Source: CAD feature listing. Evaluate the final solid. Frame: model axes, mm. Face numbers are marked on the shaded views. A direction names the side the tool comes from. Give positions to 0.01 mm unless a question says otherwise; leave off trailing zeros. Order: outer loops, then holes, each group sorted by start corner. A loop starts at its lowest first (then second) coordinate and runs counter-clockwise, first axis right, second up. Notation, with made-up numbers: (71, 33) -> (122, 33) arc R29 ccw to (122, 64) -> close; hole circle Ø7 at (37.5, -21). An arc over 180 degrees is marked (long way). Use CSV: the item, a comma, the result in double quotes.
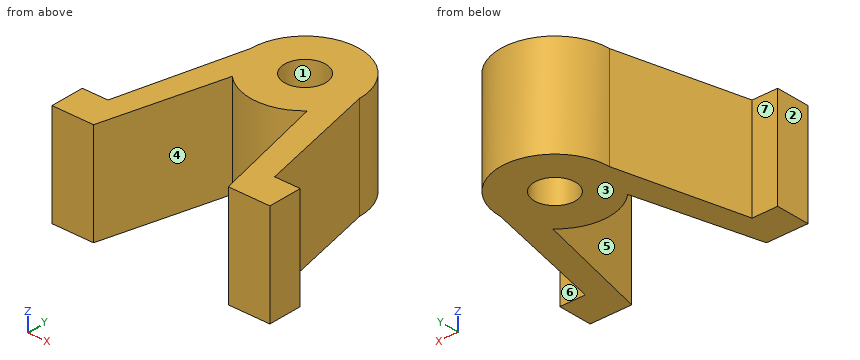
```python
from build123d import *

# Parameters (mm, degrees)
SKETCH_1_R      = 4
EXTRUDE_1_DEPTH = 20


with BuildPart() as part:
    # 草图1 → 凸台-拉伸1 (new body)
    with BuildSketch(Plane.XY):
        with BuildLine():
            Line((-37.719289559, 36.699716541), (-32.049702854, 11.94104698))
            Line((-32.049702854, 11.94104698), (-27.049702854, 11.94104698))
            Line((-27.049702854, 11.94104698), (-27.049702854, 5.329716541))
            Line((-27.049702854, 5.329716541), (-35.173631719, 5.329716541))
            Line((-35.173631719, 5.329716541), (-41.015175762, 29.009348728))
            ThreePointArc((-41.015175762, 29.009348728), (-48.339289559, 26.079716541), (-55.663403355, 29.009348728))
            Line((-55.663403355, 29.009348728), (-61.504947398, 5.329716541))
            Line((-61.504947398, 5.329716541), (-69.628876263, 5.329716541))
            Line((-69.628876263, 5.329716541), (-69.628876263, 11.94104698))
            Line((-69.628876263, 11.94104698), (-64.628876263, 11.94104698))
            Line((-64.628876263, 11.94104698), (-58.959289559, 36.699716541))
            ThreePointArc((-58.959289559, 36.699716541), (-48.339289559, 47.319716541), (-37.719289559, 36.699716541))
        make_face()
        with Locations((-48.339289559, 36.699716541)):
            Circle(SKETCH_1_R, mode=Mode.SUBTRACT)
    extrude(amount=EXTRUDE_1_DEPTH)


solid = part.part
```
1. Ray query, line 1 along X through (y, z) = (27.5, 9); line 2 along X through (y, z) = (20.5, 14.75); line 3 along X through (y, z) = (14, 12). Return the intervals inside material, ascending.
Answer below:
line 1,"x = -61.07 to -56.04, -53.64 to -43.03, -40.64 to -35.61"
line 2,"x = -62.67 to -57.76, -38.92 to -34.01"
line 3,"x = -64.16 to -59.37, -37.31 to -32.52"
2. Access query for the marked faces 5, 6 and 7. Directions: +Z, -Z, +X, -X, +Y, -Y. A direction counts if a zero-diameter tool reaches every point of the face in a straight line with its end or side. Return the directions, or none.
Answer below:
face 5,"+Z, -Z, -Y"
face 6,"+Z, -Z, +X, +Y"
face 7,"+Z, -Z, -X, +Y"
3. Section query C-C on y = 27. Return loops of the section in (x, z), plus the area to 3 significant figures.
Answer below:
outline,"(-61.18, 0) -> (-56.16, 0) -> (-56.16, 20) -> (-61.18, 20) -> close; (-52.66, 0) -> (-44.01, 0) -> (-44.01, 20) -> (-52.66, 20) -> close; (-40.52, 0) -> (-35.5, 0) -> (-35.5, 20) -> (-40.52, 20) -> close"
area,"374 mm²"
4. Pin query (flat end, axial travel): P1, Ø6, axis at x = -54, z = 15.5, coming from the +Y side; P2, Ø4, axis at x = -43.5, z = 11.5, coming from the -Y side; P3, Ø1.5, axis at y = 25, z = 9.5, coming from the +X side; P4, Ø10, axis at y = 12, z = 16, coming from the -X side. Return the tip coordinate at first contact, or that it passes through.
Answer below:
P1,"stops at y = 46.98"
P2,"stops at y = 26.47"
P3,"stops at x = -34.87"
P4,"stops at x = -69.63"
5. Section query A-A on z = 12.5. Return loops of the section in (x, y), plus the area to 3 significant figures.
Answer below:
outline,"(-69.63, 5.33) -> (-61.5, 5.33) -> (-55.66, 29.01) arc R10.62 ccw to (-41.02, 29.01) -> (-35.17, 5.33) -> (-27.05, 5.33) -> (-27.05, 11.94) -> (-32.05, 11.94) -> (-37.72, 36.7) arc R10.62 ccw to (-58.96, 36.7) -> (-64.63, 11.94) -> (-69.63, 11.94) -> close; hole circle Ø8 at (-48.34, 36.7)"
area,"619 mm²"
6. Section query B-B on x = -50. Return loops of the section in (y, z), plus the area to 3 significant figures.
Answer below:
outline,"(26.21, 0) -> (33.06, 0) -> (33.06, 20) -> (26.21, 20) -> close; (40.34, 0) -> (47.19, 0) -> (47.19, 20) -> (40.34, 20) -> close"
area,"274 mm²"
7. Mould query, pull axis X, two halves, no side actions, for the marked faces 1, 2, 3 and 4. Classes: released by +X, released by -X, zero draft, split by the parting line, or undercut.
Answer below:
face 1,"undercut"
face 2,"released by -X"
face 3,"zero draft"
face 4,"undercut"
8. Section query D-D on y = 38.5. Return loops of the section in (x, z), plus the area to 3 significant figures.
Answer below:
outline,"(-58.81, 0) -> (-51.91, 0) -> (-51.91, 20) -> (-58.81, 20) -> close; (-44.77, 0) -> (-37.87, 0) -> (-37.87, 20) -> (-44.77, 20) -> close"
area,"276 mm²"
